Could you check a few things on this model? Use its own coordinates, in mm. A direction names the side the tool comes from. Coordinates: 2 decimals unless noted, no trailing zeros. Loops run counter-clockwise (first coordinate to the right, second up) from the corner with the lowest first, then second, coordinate; pieces in that order, holes last. Notation, with made-up numbers: (71, 26) - (95, 26) arc R4 cw to (95, 30) - close; hole circle Ø4 at (-5.5, 86). An arc over 180 degrees is marked (long way). Put each result on its own line as item: value. Start each with the question number.
```python
from build123d import *
from OCP.BRepAlgoAPI import BRepAlgoAPI_Cut
from OCP.TopTools import TopTools_ListOfShape

# Parameters (mm, degrees)
SKETCH1_R           = 2.5
BOSS_EXTRUDE1_DEPTH = 190.5
FILLET1_R           = 1.5
SKETCH2_W           = 16.94037733
SKETCH2_H           = 0.5
CUT_EXTRUDE1_DEPTH  = 23
SKETCH3_R           = 2
CUT_EXTRUDE2_DEPTH  = 23


with BuildPart() as part:
    # Sketch1 → Boss-Extrude1 (new body)
    with BuildSketch(Plane.XY):
        Polygon((-1.499992211, 10), (2.38e-06, 10), (1.500001785, 10), (6.400001785, 10), (6.400001785, 9.479132912), (6.925001785, 9.479132912), (6.925001785, 8.2), (4.695347664, 8.2), (4.695347664, 6.8), (7.595347664, 3.9), (12.404655907, 3.9), (15.304655907, 6.94037733), (15.304655907, 8.199999348), (13.075001785, 8.199999348), (13.075001785, 9.565762703), (13.497472172, 9.573136951), (13.497472172, 9.999999348), (18.397472172, 9.999999348), (20.000001785, 10), (20.000001785, 8.503508491), (20.000001785, 8.500000005), (20.000001785, 3.600001911), (19.479137611, 3.600002038), (19.479137484, 3.075002038), (18.200004571, 3.075002348), (18.200005113, 5.30465647), (16.800005113, 5.30465681), (13.900004408, 2.404657514), (13.900003241, -2.404650729), (16.940379867, -5.304651467), (18.200002536, -5.304651773), (18.200003078, -3.074997652), (19.565766433, -3.074997983), (19.573140578, -3.497468372), (20.000002975, -3.497468476), (20.000001785, -8.397468476), (20.000001785, -10), (18.500003987, -10), (13.600003987, -9.99999881), (13.600004114, -9.479131722), (13.075004114, -9.479131595), (13.075004424, -8.199998683), (15.304655907, -8.199999224), (15.304655907, -6.8), (12.404655907, -3.9), (7.595347664, -3.9), (4.695347664, -6.94037733), (4.695347664, -8.2), (6.925001785, -8.2), (6.925001785, -9.565763355), (6.502531399, -9.573137603), (6.502531399, -10), (1.602531399, -10), (2.38e-06, -10), (-1.602527233, -10), (-6.502525798, -10), (-6.502525798, -9.573137078), (-6.92499762, -9.565763355), (-6.92499762, -8.2), (-4.695343498, -8.2), (-4.695343498, -6.94037733), (-7.595343498, -3.9), (-12.404651741, -3.9), (-15.304651741, -6.8), (-15.304651741, -8.2), (-13.07499762, -8.2), (-13.07499762, -9.479132912), (-13.600001017, -9.479132912), (-13.600001017, -10), (-18.49999954, -10), (-19.99999762, -10), (-19.99999762, -3.497471822), (-19.573134698, -3.497471822), (-19.565760974, -3.075), (-18.19999762, -3.075), (-18.19999762, -5.304654122), (-16.94037495, -5.304654122), (-13.89999762, -2.404654122), (-13.89999762, 2.404654122), (-16.79999762, 5.304654122), (-18.19999762, 5.304654122), (-18.19999762, 3.075), (-19.479130532, 3.075), (-19.479130532, 3.600003398), (-19.99999762, 3.600003398), (-19.99999762, 10), (-13.497469442, 10), (-13.497469442, 9.573137078), (-13.07499762, 9.565763355), (-13.07499762, 8.2), (-15.304651741, 8.2), (-15.304651741, 6.94037733), (-12.404651741, 3.9), (-7.595343498, 3.9), (-4.695343498, 6.8), (-4.695343498, 8.2), (-6.92499762, 8.2), (-6.92499762, 9.479132912), (-6.399994222, 9.479132912), (-6.399994222, 10), align=None)
        with Locations((-9.99999762, 0)):
            Circle(SKETCH1_R, mode=Mode.SUBTRACT)
        with Locations(Location((9.99999762, 0, 0), (0, 0, 180))):
            Circle(SKETCH1_R, mode=Mode.SUBTRACT)
        Polygon((-3.059620289, 5.304654122), (-3.059620289, 8.2), (2.38e-06, 8.2), (3.059624455, 8.2), (3.059624455, 5.304654122), (6.100001785, 2.404654122), (6.100001785, -2.404654122), (3.200001785, -5.304654122), (3.200001785, -8.2), (2.38e-06, -8.2), (-3.19999762, -8.2), (-3.19999762, -5.304654122), (-6.09999762, -2.404654122), (-6.09999762, 2.404654122), align=None, mode=Mode.SUBTRACT)
    extrude(amount=-BOSS_EXTRUDE1_DEPTH)

    # Fillet1
    fillet1_edges = [part.edges().sort_by_distance(p)[0] for p in [
        (20.000001785, 10, -95.25),
        (20.000001785, -10, -95.25),
        (-19.99999762, -10, -95.25),
        (-19.99999762, 10, -95.25),
    ]]
    fillet(fillet1_edges, radius=FILLET1_R - 0.0001)  # a hair under: the kernel refuses the full size


with BuildPart() as cut_extrude1_tool:
    # Sketch2 → Cut-Extrude1 (new body)
    with BuildSketch(Plane(origin=(0, 10, 0), x_dir=(1, 0, 0), z_dir=(0, 1, 0))):
        with Locations((11.52981312, 190.25)):
            Rectangle(SKETCH2_W, SKETCH2_H)
    extrude(amount=-CUT_EXTRUDE1_DEPTH)


with BuildPart() as part_1:
    add(part.part)

    # Cut-Extrude1: cut by cut_extrude1_tool, with a tolerance
    cut_extrude1_stock = TopTools_ListOfShape()
    cut_extrude1_stock.Append(part_1.part.wrapped)
    cut_extrude1_tools = TopTools_ListOfShape()
    cut_extrude1_tools.Append(cut_extrude1_tool.part.wrapped)
    cut_extrude1_cut = BRepAlgoAPI_Cut()
    cut_extrude1_cut.SetArguments(cut_extrude1_stock)
    cut_extrude1_cut.SetTools(cut_extrude1_tools)
    cut_extrude1_cut.SetFuzzyValue(0.00001)
    cut_extrude1_cut.Build()
    add(Compound.cast(cut_extrude1_cut.Shape()).solids(), mode=Mode.REPLACE)

    # Sketch3 → Cut-Extrude2 (cut)
    with BuildSketch(Plane.XZ.offset(10)):
        with Locations(Location((2.8e-06, -148.5, 0), (0, 0, 270))):
            Circle(SKETCH3_R)
    extrude(amount=-CUT_EXTRUDE2_DEPTH, mode=Mode.SUBTRACT)


solid = part_1.part
```
(1) For pin 1 Ø0.6 at (x, z) = (19, -77) entering from -Y; pin 2 Ø5 at (x, y) = (8.5, 0) entering from -Z; pin 3 Ø5.5 at (x, z) = (10.5, -126) entering from -Y, each with a flat end and sliding along its axis, tell me the tip position at first contact or that it passes through.
(2) I want a section at B-B on z = -148.5. Count the separate pieces of the cut face and the enclosed holes in it, and give its area (3 significant figures).
(3) I need wall thicknesses on L1, parallel to X at y = -7.75, z = -166; L2, parallel to Y at x = -3, z = -29.5; L3, parallel to X at y = 8, z = -91.5. Which ranges of each line are inside material? Lowest first, please. Write a range as [from, to].
(4) Which directions (+Z, -Z, +X, -X, +Y, -Y) give clear straight access to the entire face, cutting with the end or side of a thin tool? Please do faces 4 (the cylindrical face through (0.088, 9.087, -146.502)), 5 (the flat face through (-6.125, -5.441, -93.916)), 6 (the flat face through (10, 3.9, -94)).
(5) I want a section at A-A on y = 0. List the corners of the cut face in (x, z) for me.
(6) If we mould it in two halves opening along X, with no side actions, what happens to faces 1 (the flat face through (13, 0, -190)), 2 (the flat face through (13.9, 0, -94)), 3 (the flat face through (-13.875, 5.441, -93.916))? For each: pulls with the +X half, pulls with the -X half, needs draft (parallel to the pull), parting line crosses it, or undercut.
Answer sheet:
1. pin 1: stops at y = -9.99
1. pin 2: stops at z = -190
1. pin 3: stops at y = -9.48
2. separate pieces: 2
2. enclosed holes: 2
2. area: 305 mm^2
3. L1: x = [-20, -15.3], [-4.7, -3.2], [3.2, 4.7], [15.3, 20]
3. L2: y = [-10, -8.2], [8.2, 10]
3. L3: x = [-20, -15.3], [-4.7, -3.06], [3.06, 4.7], [15.3, 20]
4. face 4: +Y, -Y
4. face 5: +Z, -Z
4. face 6: +Z, -Z, +Y
5. outline: (-13.9, -190.5) - (-12.5, -190.5) - (-12.5, 0) - (-13.9, 0) - close; (-7.5, -190.5) - (-6.1, -190.5) - (-6.1, 0) - (-7.5, 0) - close; (6.1, -190) - (7.5, -190) - (7.5, 0) - (6.1, 0) - close; (12.5, -190) - (13.9, -190) - (13.9, 0) - (12.5, 0) - close
6. face 1: needs draft
6. face 2: pulls with the +X half
6. face 3: undercut
